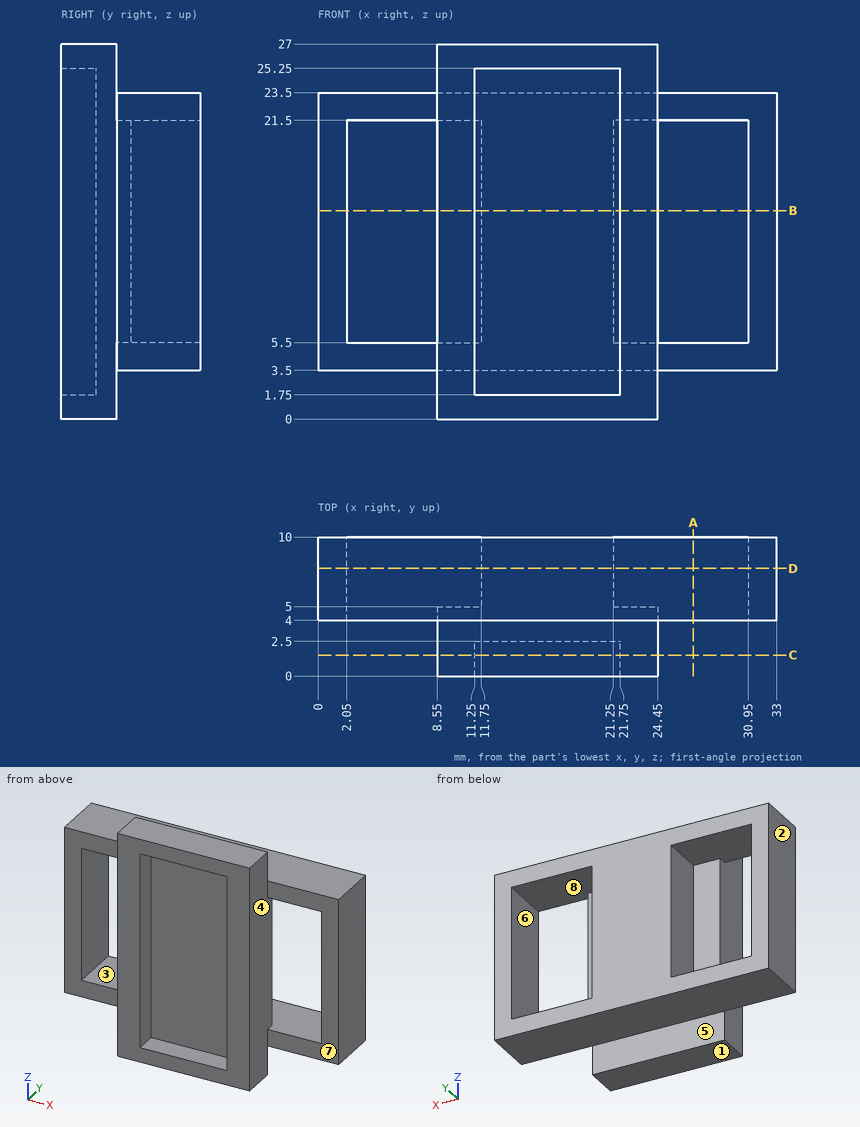
Job drawing, mm, ordinate dimensions from the low corner. One solid piece. A direction names the side the tool comes from. Give positions to 0.01 mm unless a question says otherwise; leave off trailing zeros. Order: outer loops, then holes, each group sorted by start corner. A loop starts at its lowest first (then second) coordinate and runs counter-clockwise, first axis right, second up. Notation, with made-up numbers: (31, 79) -> (87, 79) arc R6 ccw to (87, 85) -> close; hole circle Ø9 at (79.5, 50.5). An arc over 180 degrees is marked (long way). Return JSON: item names as keys, results as strings.
Q1. Saw through at C-C (y = 1.5). Write the cut outline in (x, z), then the cut area to 3 significant figures.
Working result:
{"outline": "(8.55, 0) -> (24.45, 0) -> (24.45, 27) -> (8.55, 27) -> close; hole (11.25, 1.75) -> (21.75, 1.75) -> (21.75, 25.25) -> (11.25, 25.25) -> close", "area": "183 mm²"}
Q2. Saw through at B-B (z = 15). Write the cut outline in (x, y).
Working result:
{"outline": "(0, 4) -> (2.05, 4) -> (2.05, 10) -> (0, 10) -> close; (8.55, 0) -> (11.25, 0) -> (11.25, 2.5) -> (21.75, 2.5) -> (21.75, 0) -> (24.45, 0) -> (24.45, 5) -> (21.25, 5) -> (21.25, 10) -> (11.75, 10) -> (11.75, 5) -> (8.55, 5) -> close; (30.95, 4) -> (33, 4) -> (33, 10) -> (30.95, 10) -> close"}
Q3. Which spindle directions (+Z, -Z, +X, -X, +Y, -Y) get a long thin tool onto all of the face, cutting with end or side? Do the marked faces 4, 5, 6, 7 and 8. Say none if no direction does.
Working result:
{"face 4": "-Y", "face 5": "-Z, +X, -X, +Y", "face 6": "+Y, -Y", "face 7": "+Z, -Z, +X, -Y", "face 8": "+Y"}
Q4. Flat gauge pins, fed straight in: pin 1 (1 mm diameter, centred on x = 15.5, z = 26, fed in from +Y); pin 2 (4.5 mm diameter, centred on x = 30.5, z = 10, fed in from -Y); pin 3 (5 mm diameter, centred on x = 15.5, z = 10, fed in from -Y). Where does each tip first touch, or does it go through?
Working result:
{"pin 1": "y = 4", "pin 2": "y = 4", "pin 3": "y = 2.5"}
Q5. Saw through at D-D (y = 7.75). Write the cut outline in (x, z).
Working result:
{"outline": "(0, 3.5) -> (33, 3.5) -> (33, 23.5) -> (0, 23.5) -> close; hole (2.05, 5.5) -> (11.75, 5.5) -> (11.75, 21.5) -> (2.05, 21.5) -> close; hole (21.25, 5.5) -> (30.95, 5.5) -> (30.95, 21.5) -> (21.25, 21.5) -> close"}
Q6. Saw through at A-A (x = 27). Write the cut outline in (y, z), then the cut area to 3 significant figures.
Working result:
{"outline": "(4, 3.5) -> (10, 3.5) -> (10, 5.5) -> (4, 5.5) -> close; (4, 21.5) -> (10, 21.5) -> (10, 23.5) -> (4, 23.5) -> close", "area": "24.0 mm²"}
Q7. Drill centre lines: line 1 (Z direction, x = 27, y = 8.5); line 2 (X direction, y = 7, z = 15.5); line 3 (X direction, y = 1.25, z = 12.25). Where is each one in solid material? Low to high.
Working result:
{"line 1": "3.5 to 5.5, 21.5 to 23.5", "line 2": "0 to 2.05, 11.75 to 21.25, 30.95 to 33", "line 3": "8.55 to 11.25, 21.75 to 24.45"}
Q8. Mould opens along X. For the marked faces 1, 2 and 3 say: pulls with the +X half, pulls with the -X half, needs draft (parallel to the pull), parting line crosses it, or undercut.
Working result:
{"face 1": "needs draft", "face 2": "pulls with the -X half", "face 3": "undercut"}
